from build123d import *

# Parameters (mm, degrees)
SKETCH_1_R      = 40
EXTRUDE_1_DEPTH = 50
SKETCH_2_R      = 40
EXTRUDE_2_DEPTH = 50
SKETCH_3_R      = 30
EXTRUDE_3_DEPTH = 62.4


with BuildPart() as part:
    # Sketch 1 → Extrude 1 (new, symmetric)
    with BuildSketch(Plane(origin=(0, 0, 0), x_dir=(0, 0, -1), z_dir=(1, 0, 0))):
        Circle(SKETCH_1_R)
    extrude(amount=EXTRUDE_1_DEPTH, both=True)



with BuildPart() as body_2:
    # Sketch 2 → Extrude 2 (new, symmetric)
    with BuildSketch(Plane(origin=(-162.4, 0, 0), x_dir=(0, 0, -1), z_dir=(1, 0, 0))):
        Circle(SKETCH_2_R)
    extrude(amount=EXTRUDE_2_DEPTH, both=True)


with BuildPart() as part_1:
    add(part.part)

    add(body_2.part)  # Extrude 3 merges body 2
    # Sketch 3 → Extrude 3 (add)
    with BuildSketch(Plane(origin=(-112.4, 0, 0), x_dir=(0, 0, -1), z_dir=(1, 0, 0))):
        Circle(SKETCH_3_R)
    extrude(amount=EXTRUDE_3_DEPTH)


solid = part_1.part
Part model, mm, in its own coordinate system. A direction names the side the tool comes from. Coordinates: 2 decimals unless noted, no trailing zeros. Write each loop counter-clockwise with the first axis right and the second up, starting at its lowest first coordinate (ties: lowest second). Pieces come first, ordered by that corner, then holes. Notation, with made-up numbers: M -22,-37.5 L 31,-37.5 A17 cw 31,-9.5 Z; hole C 22.25,88.25 d8. An arc over 180 degrees is marked long. Return JSON: item names as keys, results as strings.
1. Flat gauge pins, fed straight in: pin 1 Ø5 at (x, z) = (-140.5, 31) entering from -Y; pin 2 Ø1 at (x, z) = (-38, 6.5) entering from -Y; pin 3 Ø5 at (x, y) = (-137.5, 8.5) entering from -Z. Where does each tip first touch, or does it go through?
Determined:
{"pin 1": "y = -28.07", "pin 2": "y = -39.55", "pin 3": "z = -39.55"}
2. Pull direction X, two halves, no side cores. Call faces 3 (the face through (-50, 30, -6)), 4 (the face through (-161.7, -39.05, 8.67)), 5 (the face through (-212.4, 1, 1)), 6 (the face through (50, 1, 1)): pulls with the +X half, pulls with the -X half, needs draft (parallel to the pull), parting line crosses it, or undercut.
Determined:
{"face 3": "undercut", "face 4": "needs draft", "face 5": "pulls with the -X half", "face 6": "pulls with the +X half"}
3. Saw through at A-A, the plane z = -34. Write the cut outline in (x, y), then the cut area to 3 significant figures.
Determined:
{"outline": "M -212.4,-21.07 L -112.4,-21.07 L -112.4,21.07 L -212.4,21.07 Z; M -50,-21.07 L 50,-21.07 L 50,21.07 L -50,21.07 Z", "area": "8,430 mm²"}
4. Saw through at B-B, the plane y = 0. Write the cut outline in (x, z).
Determined:
{"outline": "M -212.4,-40 L -112.4,-40 L -112.4,-30 L -50,-30 L -50,-40 L 50,-40 L 50,40 L -50,40 L -50,30 L -112.4,30 L -112.4,40 L -212.4,40 Z"}
5. Probe L1, parallel to X at y = -27, z = 20.5; L2, parallel to Y at x = -160.5, z = 0.5; L3, parallel to Y at x = -146.5, z = 28.5. List the from-to ranges inside material, lowest first.
Determined:
{"L1": "-212.4 to -112.4, -50 to 50", "L2": "-40 to 40", "L3": "-28.07 to 28.07"}
6. 3-axis set-ups, long thin cutter, end or side, ignore diameter. For faces 1 (the face through (0.7, -39.05, 8.67)), 2 (the face through (-81.64, 1.32, 29.97)): which of +Z, -Z, +X, -X, +Y, -Y reach the whole face in a straight line?
Determined:
{"face 1": "+X, -X", "face 2": "none"}
7. Saw through at D-D, the plane x = -10.5. Write the cut outline in (y, z), then the cut area to 3 significant figures.
Determined:
{"outline": "C 0,0 d80", "area": "5,030 mm²"}
